For this review, take the finished solid that the model builds, in its own axes (mm). Give positions to 0.01 mm unless a question says otherwise; leave off trailing zeros. Write each loop counter-clockwise with the first axis right and the second up, starting at its lowest first coordinate (ties: lowest second). Pieces come first, ordered by that corner, then holes.
1) Wall thickness on line 1 along Y through (x, z) = (166.5, 1); line 2 along X through (y, z) = (-317, 5.5); line 3 along X through (y, z) = (-159, 6.25): over which ranges is each line inside the solid? List them lowest first.
2) For P1, Ø1.5, axis at y = -56.5, z = 4.5, coming from the +X side, flat-tipped, find the tip position at first contact; note if it passes through.
3) We need section A-A on y = -244. Give the boundary of the cut face in (x, z).
4) We need section B-B on z = 4.25. Give the boundary of the cut face in (x, y).
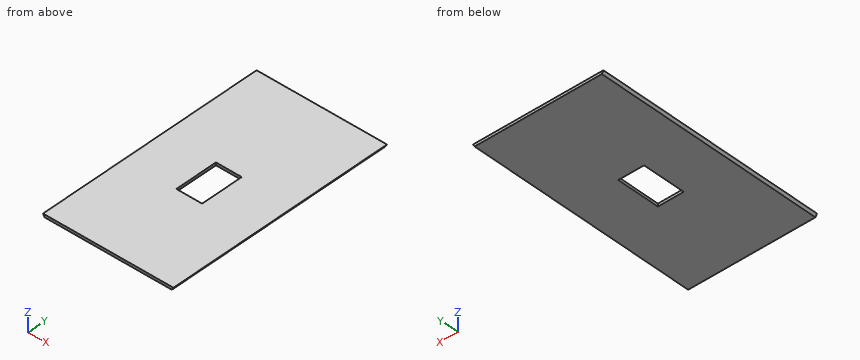
Autodesk Inventor part; units mm, degrees
ref_plane "YZ Plane" through (0, 0, 0) normal (1, 0, 0) x (0, 1, 0)
ref_plane "XZ Plane" through (0, 0, 0) normal (0, 1, 0) x (-1, 0, 0)
ref_plane "XY Plane" through (0, 0, 0) normal (0, 0, 1) x (1, 0, 0)
sketch "Sketch1" plane through (0, 0, 0) normal (0, 0, 1) x (1, 0, 0)
  line L0 (0, 0) -> (303.5592, 0)
  line L1 (303.5592, 0) -> (303.5592, -533.4)
  line L2 (303.5592, -533.4) -> (0, -533.4)
  line L3 (0, -533.4) -> (0, 0)
  line L4 (455.3388, 262.89) -> (303.5592, 0)
  line L5 (303.5592, 0) -> (0, 0)
  line L6 (0, 0) -> (-151.7796, 262.89)
  line L7 (-151.7796, 262.89) -> (0, 525.78)
  line L8 (0, 525.78) -> (303.5592, 525.78)
  line L9 (303.5592, 525.78) -> (455.3388, 262.89)
  point P0 (151.7796, 262.89)
  dimension "d1" = 533.4
  dimension "d54" = 525.78
extrude "Extrusion1" add sketch "Sketch1" along normal blind 6.35 contours L0 L1 L2 L3
sketch "Sketch2" plane through (0, 0, 0) normal (0, 1, 0) x (1, 0, 0)
  line L0 (303.5592, -6.35) -> (0, -6.35)
  line L1 (0, -6.35) -> (-3.6662, -6.35)
  line L2 (-3.6662, -6.35) -> (0, 0)
  line L3 (0, 0) -> (0, -6.35)
  line L4 (0, 0) -> (0, -6.35)
  line L5 (0, -6.35) -> (0, 0)
  line L6 (303.5592, -6.35) -> (307.2254, -6.35)
  line L7 (303.5592, 0) -> (303.5592, -6.35)
  line L8 (307.2254, -6.35) -> (303.5592, 0)
  line L9 (303.5592, 0) -> (303.5592, -6.35)
  dimension "d4" = 30
  dimension "d5" = 60
extrude "Extrusion2" add sketch "Sketch2" against normal blind 533.4
sketch "Sketch4" plane through (0, 0, 6.35) normal (0, 0, 1) x (1, 0, 0)
  line L0 (137.7796, -228.6) -> (165.7796, -228.6)
  line L1 (165.7796, -228.6) -> (165.7796, -278.6)
  line L2 (165.7796, -278.6) -> (137.7796, -278.6)
  line L3 (137.7796, -278.6) -> (137.7796, -228.6)
  line L4 (-3.6662, 0) -> (-3.6662, -533.4)
  line L5 (-3.6662, 0) -> (307.2254, 0)
  line L6 (307.2254, -533.4) -> (-3.6662, -533.4)
  circle A0 centre (131.7796, -253.6) radius 3
  circle A1 centre (171.7796, -253.6) radius 3
  point P0 (0, 0)
  point P1 (151.7796, -228.6)
  point P2 (151.7796, 0)
  point P3 (165.7796, -253.6)
  point P4 (137.7796, -253.6)
  dimension "d16" = 28
  dimension "d17" = 50
  dimension "d19" = 6
  dimension "d20" = 6
  dimension "d21" = 6
  dimension "d22" = 6
  dimension "d41" = 228.6
extrude "Extrusion4" cut sketch "Sketch4" against normal through all
sketch "Sketch5" plane through (0, 0, 6.35) normal (0, 0, 1) x (1, 0, 0)
  line L0 (195.2796, -309.6) -> (108.2796, -309.6)
  line L1 (108.2796, -309.6) -> (108.2796, -298.6)
  line L2 (108.2796, -298.6) -> (195.2796, -298.6)
  line L3 (195.2796, -298.6) -> (195.2796, -309.6)
  line L4 (165.7796, -278.6) -> (137.7796, -278.6)
  line L5 (181.2796, -330.6) -> (159.2796, -330.6)
  line L6 (159.2796, -330.6) -> (159.2796, -318.6)
  line L7 (159.2796, -318.6) -> (181.2796, -318.6)
  line L8 (181.2796, -318.6) -> (181.2796, -330.6)
  line L9 (144.2796, -334.6) -> (122.2796, -334.6)
  line L10 (122.2796, -334.6) -> (122.2796, -314.6)
  line L11 (122.2796, -314.6) -> (144.2796, -314.6)
  line L12 (144.2796, -314.6) -> (144.2796, -334.6)
  line L13 (159.2796, -324.6) -> (144.2796, -324.6) construction
  point P0 (0, 0)
  point P1 (151.7796, -298.6)
  point P2 (151.7796, -278.6)
  point P3 (151.7796, -324.6)
  dimension "d26" = 87
  dimension "d27" = 11
  dimension "d28" = 20
  dimension "d29" = 22
  dimension "d30" = 12
  dimension "d32" = 22
  dimension "d33" = 20
  dimension "d37" = 15
  dimension "d38" = 15
extrude "Extrusion5" cut sketch "Sketch5" against normal through all
sketch "Sketch7" plane through (0, 0, 6.35) normal (0, 0, 1) x (1, 0, 0)
  line L0 (101.7796, -345) -> (201.7796, -345)
  line L1 (201.7796, -345) -> (201.7796, -225)
  line L2 (201.7796, -225) -> (101.7796, -225)
  line L3 (101.7796, -225) -> (101.7796, -345)
  line L4 (-3.6662, 0) -> (307.2254, 0)
  point P0 (0, 0)
  point P1 (151.7796, -225)
  point P2 (151.7796, 0)
  dimension "d49" = 100
  dimension "d50" = 120
  dimension "d51" = 225
extrude "Extrusion7" cut sketch "Sketch7" against normal through all
sketch "Sketch8" plane through (0, 0, 0) normal (0, 1, 0) x (1, 0, 0)
  line L0 (-3.6662, -6.35) -> (307.2254, -6.35)
  line L1 (0, 0) -> (-3.6662, 0)
  line L2 (-3.6662, 0) -> (-3.6662, -6.35)
  line L3 (-3.6662, -6.35) -> (0, -6.35)
  line L4 (0, -6.35) -> (0, 0)
  line L5 (0, 0) -> (303.5592, 0)
  line L6 (307.2254, -6.35) -> (303.5592, -6.35)
  line L7 (303.5592, -6.35) -> (303.5592, 0)
  line L8 (303.5592, 0) -> (307.2254, 0)
  line L9 (307.2254, 0) -> (307.2254, -6.35)
extrude "Extrusion8" cut sketch "Sketch8" against normal through all contours L2 L1 L4 L0 | L7 L8 L9 L0
sketch "Sketch9" plane through (0, 0, 6.35) normal (0, 0, 1) x (1, 0, 0)
  line L0 (121.7796, -335) -> (181.7796, -335)
  line L1 (181.7796, -335) -> (181.7796, -235)
  line L2 (181.7796, -235) -> (121.7796, -235)
  line L3 (121.7796, -235) -> (121.7796, -335)
  line L4 (0, 0) -> (303.5592, 0)
  line L5 (101.7796, -345) -> (101.7796, -225)
  line L6 (201.7796, -225) -> (201.7796, -345)
  line L7 (201.7796, -345) -> (101.7796, -345)
  line L8 (101.7796, -345) -> (101.7796, -225)
  line L9 (101.7796, -225) -> (201.7796, -225)
  line L10 (0, 0) -> (0, -533.4)
  line L11 (303.5592, -533.4) -> (0, -533.4)
  line L12 (303.5592, -533.4) -> (303.5592, 0)
  line L13 (0, 0) -> (303.5592, 0)
  point P0 (121.7796, -285)
  point P1 (101.7796, -285)
  point P2 (151.7796, -235)
  point P3 (151.7796, 0)
  dimension "d57" = 60
  dimension "d58" = 100
extrude "Extrusion9" add sketch "Sketch9" against normal blind 6.35 contours L5 L9 L6 L7
sketch "Sketch10" plane through (0, 0, 6.35) normal (0, 0, 1) x (1, 0, 0)
  line L0 (0, -533.4) -> (0, 0)
  line L1 (0, -533.4) -> (303.5592, -533.4)
  line L2 (303.5592, -533.4) -> (303.5592, -539.75)
  line L3 (303.5592, -539.75) -> (0, -539.75)
  line L4 (0, -539.75) -> (0, -533.4)
  dimension "d61" = 6.35
extrude "Extrusion10" add sketch "Sketch10" against normal blind 6.35
sketch "Sketch11" plane through (0, 0, 0) normal (0, 1, 0) x (1, 0, 0)
  line L0 (0, -6.35) -> (303.5592, -6.35) construction
  line L1 (0, -6.35) -> (3.6662, 0)
  line L2 (0, 0) -> (303.5592, 0) construction
  line L3 (3.6662, 0) -> (0, 0)
  line L4 (0, 0) -> (0, -6.35)
  line L5 (303.5592, -6.35) -> (299.8931, 0)
  line L6 (299.8931, 0) -> (303.5592, 0)
  line L7 (303.5592, -6.35) -> (303.5592, 0)
  line L8 (303.5592, -6.35) -> (303.5592, 0)
  dimension "d64" = 30
  dimension "d65" = 30
extrude "Extrusion11" cut sketch "Sketch11" against normal through all
properties part number "BA03" material "ABS Plastic"
Results list:
1. line 1: y = -539.75 to -335, -235 to 0
1. line 2: x = 0.49 to 121.78, 181.78 to 303.07
1. line 3: x = 0.06 to 303.5
2. P1: stops at x = 302.92
3. outline: (0, 6.35) - (3.67, 0) - (121.78, 0) - (121.78, 6.35) - close; (181.78, 0) - (299.89, 0) - (303.56, 6.35) - (181.78, 6.35) - close
4. outline: (1.21, -539.75) - (302.35, -539.75) - (302.35, 0) - (1.21, 0) - close; hole (121.78, -335) - (181.78, -335) - (181.78, -235) - (121.78, -235) - close
